Build history of the part. All positions in model axes, mm. Face numbers are marked on the shaded views. A direction names the side the tool comes from. Give positions to 0.01 mm unless a question says otherwise; leave off trailing zeros. Order: outer loops, then holes, each group sorted by start corner. A loop starts at its lowest first (then second) coordinate and runs counter-clockwise, first axis right, second up. Notation, with made-up numbers: M 4,-30.75 L 51,-30.75 A35 cw 51,7.25 Z; hole C -8,80.5 d3. An arc over 180 degrees is marked long. One line per item, written item: value.
from build123d import *

# Parameters (mm, degrees)
SKETCH_1_W      = 28
SKETCH_1_H      = 3
EXTRUDE_1_DEPTH = 10
FILLET_1_R      = 3
FILLET_2_R      = 0.5


with BuildPart() as part:
    # Эскиз1 → Бобышка-Вытянуть1 (new body)
    with BuildSketch(Plane(origin=(0, 0, 0), x_dir=(1, 0, 0), z_dir=(0, 1, 0))):
        with BuildLine():
            ThreePointArc((-25.941942596, 6.415014515), (-7.956456947, 7.015014515), (10.029028702, 6.415014515))
            ThreePointArc((10.029028702, 6.415014515), (10.229028702, 0.915014515), (10.029028702, -4.584985485))
            ThreePointArc((10.029028702, -4.584985485), (-7.970971298, -5.184985485), (-25.970971298, -4.584985485))
            ThreePointArc((-25.970971298, -4.584985485), (-26.141942596, 0.915504007), (-25.941942596, 6.415014515))
        make_face()
        with Locations((-7.970971298, 0.915014515)):
            Rectangle(SKETCH_1_W, SKETCH_1_H, mode=Mode.SUBTRACT)
    extrude(amount=EXTRUDE_1_DEPTH)

    # Скругление1
    fillet_1_edges = [part.edges().sort_by_distance(p)[0] for p in [
        (-25.941942596, 5, -6.415014515),
        (10.029028702, 5, -6.415014515),
        (10.029028702, 5, 4.584985485),
        (-25.970971298, 5, 4.584985485),
    ]]
    fillet(fillet_1_edges, radius=FILLET_1_R)

    # Скругление2
    fillet_2_edges = [part.edges().sort_by_distance(p)[0] for p in [
        (-21.970971298, 5, -2.415014515),
        (-21.970971298, 5, 0.584985485),
        (6.029028702, 5, 0.584985485),
        (6.029028702, 5, -2.415014515),
    ]]
    fillet(fillet_2_edges, radius=FILLET_2_R)


solid = part.part
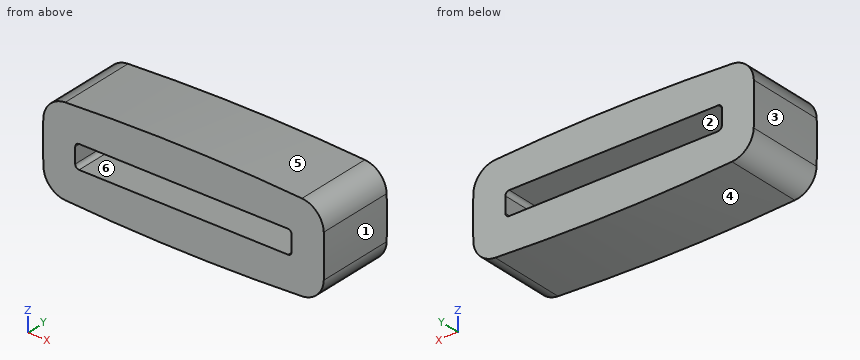
1) Tool access for the marked faces 1, 2 and 3: list every direction of +Z, -Z, +X, -X, +Y, -Y with a clear straight run to the whole face (end or side of a thin tool).
Check values:
face 1: +X, +Y, -Y
face 2: +Y, -Y
face 3: -X, +Y, -Y
2) Mould opens along Z. For the marked faces 4, 5 and 6 say: released by +Z, released by -Z, zero draft, split by the parting line, or undercut.
Check values:
face 4: released by -Z
face 5: released by +Z
face 6: undercut
3) Saw through at B-B, the plane x = -4. Write the cut outline in (y, z), then the cut area to 3 significant figures.
Check values:
outline: M 0,-6.99 L 10,-6.99 L 10,-2.42 L 0,-2.42 Z; M 0,0.58 L 10,0.58 L 10,5.16 L 0,5.16 Z
area: 91.4 mm^2
4) Drill centre lines: probe 1 along X at (y, z) = (2.5, -1.25); probe 2 along X at (y, z) = (7, 0.25); probe 3 along Z at (x, y) = (-0.5, 9). Where is each one in solid material? Low to high. Write a range as from..to.
Check values:
probe 1: -26.14..-21.97, 6.03..10.23
probe 2: -26.14..-21.94, 6..10.22
probe 3: -6.91..-2.42, 0.58..5.08
5) Saw through at A-A, the plane x = -13.5. Write the cut outline in (y, z), then the cut area to 3 significant figures.
Check values:
outline: M 0,-6.96 L 10,-6.96 L 10,-2.42 L 0,-2.42 Z; M 0,0.58 L 10,0.58 L 10,5.13 L 0,5.13 Z
area: 90.9 mm^2
6) Pin check, flat tips, straight feed: pin 1 (1 mm diameter, centred on y = 4.5, z = 2, fed in from +X); pin 2 (4 mm diameter, centred on x = 3.5, y = 3.5, fed in from -Z); pin 3 (1 mm diameter, centred on x = -12, z = -1, fed in from +Y). Stop position of each tip, or through.
Check values:
pin 1: x = 10.19
pin 2: z = -6.85
pin 3: through
